Can you work these out from the model? Positions are in its coordinate system, mm. Round coordinates to 2 decimals unless told otherwise and drop trailing zeros. Loops run counter-clockwise (first coordinate to the right, second up) from the corner with the lowest first, then second, coordinate; pieces in that order, holes last. Notation, with made-up numbers: (38, 5) -> (89, 5) arc R33 cw to (89, 34) -> close; hole circle Ø6 at (6, -27.5). An arc over 180 degrees is marked (long way). Write each question's results on one line, items separated by ' | '.
Autodesk Inventor part; units mm, degrees
ref_plane "YZ Plane" through (0, 0, 0) normal (1, 0, 0) x (0, 1, 0)
ref_plane "XZ Plane" through (0, 0, 0) normal (0, 1, 0) x (-1, 0, 0)
ref_plane "XY Plane" through (0, 0, 0) normal (0, 0, 1) x (1, 0, 0)
sketch "Sketch1" plane through (0, 0, 0) normal (0, 1, 0) x (-1, 0, 0)
  line L0 (0, -83) -> (62.9285, -83)
  line L1 (0, -83) -> (-62.9285, -83)
  line L2 (0, -73) -> (59.3296, -73)
  line L3 (0, -73) -> (-59.3296, -73)
  arc A0 (65.4207, -82.1287) -> (-65.4207, -82.1287) centre (0, 0) ccw
  arc A1 (61.9375, -72.033) -> (-61.9375, -72.033) centre (0, 0) ccw
  arc A2 (59.3296, -73) -> (61.9375, -72.033) centre (59.3296, -69) ccw
  arc A3 (62.9285, -83) -> (65.4207, -82.1287) centre (62.9285, -79) ccw
  arc A4 (-65.4207, -82.1287) -> (-62.9285, -83) centre (-62.9285, -79) ccw
  arc A5 (-61.9375, -72.033) -> (-59.3296, -73) centre (-59.3296, -69) ccw
  circle A6 centre (55.557, 83.147) radius 1.6
  circle A7 centre (-55.557, 83.147) radius 1.6
  circle A8 centre (54.3117, -78) radius 1.6
  circle A9 centre (-54.3117, -78) radius 1.6
  point P0 (64.3117, -83)
  point P1 (-64.3117, -83)
  point P2 (60.7947, -73)
  point P3 (-60.7947, -73)
  dimension "d3" = 10
  dimension "d6" = 3.2
  dimension "d9" = 3.2
  dimension "d10" = 3.2
extrude "Extrusion1" add sketch "Sketch1" along normal blind 2
properties part number "Handle Ring"
1. If we section it at B-B (z = 0): List the corners of the cut face in (x, y) for me.
Final values:
outline: (-105, 0) -> (-95, 0) -> (-95, 2) -> (-105, 2) -> close; (95, 0) -> (105, 0) -> (105, 2) -> (95, 2) -> close
2. Please list where these lines run through material, in increasing order: line 1 (Z direction, x = 0, y = 0.8); line 2 (Z direction, x = -74, y = 1.55); line 3 (X direction, y = 1, z = -57.5). Write a range as from..to.
Final values:
line 1: -83..-73, 95..105 | line 2: -74.49..-59.57, 59.57..74.49 | line 3: -87.86..-75.62, 75.62..87.86
3. Will this pin go through, and if not, where does the flat tip stop? pin 1 (0.6 mm diameter, centred on x = -24, y = 1, fed in from +Z).
Final values:
pin 1: z = 102.29
4. If we section it at C-C (y = 1.1): List the corners of the cut face in (x, z) for me, then the cut area to 3 significant figures.
Final values:
outline: (-65.42, -82.13) arc R4 ccw to (-62.93, -83) -> (62.93, -83) arc R4 ccw to (65.42, -82.13) arc R105 ccw (long way) to start; hole (-61.94, -72.03) arc R4 ccw to (-59.33, -73) -> (59.33, -73) arc R4 ccw to (61.94, -72.03) arc R95 ccw (long way) to start; hole circle Ø3.2 at (-55.56, 83.15); hole circle Ø3.2 at (-54.31, -78); hole circle Ø3.2 at (54.31, -78); hole circle Ø3.2 at (55.56, 83.15) | area: 6,150 mm2
5. If we section it at A-A (x = 0): List the corners of the cut face in (y, z) for me, then the cut area to 3 significant figures.
Final values:
outline: (0, -83) -> (2, -83) -> (2, -73) -> (0, -73) -> close; (0, 95) -> (2, 95) -> (2, 105) -> (0, 105) -> close | area: 40.0 mm2
